Geometry check sheet. Reference: the model listing, model coordinates, mm. Coordinates: 2 decimals unless noted, no trailing zeros. Loops run counter-clockwise (first coordinate to the right, second up) from the corner with the lowest first, then second, coordinate; pieces in that order, holes last. Notation, with made-up numbers: M 79,85 L 118,85 A31 cw 118,121 Z; hole C -3,18.25 d5. An arc over 180 degrees is marked long. Use CSV: the item, a comma, the result in double quotes.
```python
from build123d import *

# Parameters (mm, degrees)
F0_R     = 11
F1_DEPTH = 6


with BuildPart() as f1:
    # F0 (on Top) → F1 (new body)
    with BuildSketch(Plane.XY):
        with BuildLine():
            ThreePointArc((36.158809, 0), (25.158809, 11), (14.158809, 0))
            ThreePointArc((14.158809, 0), (25.158809, -11), (36.158809, 0))
        make_face()
        with Locations((-25.158809, 0)):
            Circle(F0_R)
        with BuildLine():
            ThreePointArc((5.524196, 13.945725), (0, 37.658809), (-5.524196, 13.945725))
            ThreePointArc((-5.524196, 13.945725), (-8.236389, 12.536423), (-10.606602, 10.606602))
            ThreePointArc((-10.606602, 10.606602), (-12.536423, 8.236389), (-13.945725, 5.524196))
            ThreePointArc((-13.945725, 5.524196), (-37.658809, 0), (-13.945725, -5.524196))
            ThreePointArc((-13.945725, -5.524196), (-12.536423, -8.236389), (-10.606602, -10.606602))
            ThreePointArc((-10.606602, -10.606602), (-8.236389, -12.536423), (-5.524196, -13.945725))
            ThreePointArc((-5.524196, -13.945725), (0, -37.658809), (5.524196, -13.945725))
            ThreePointArc((5.524196, -13.945725), (8.236389, -12.536423), (10.606602, -10.606602))
            ThreePointArc((10.606602, -10.606602), (12.536423, -8.236389), (13.945725, -5.524196))
            ThreePointArc((13.945725, -5.524196), (37.658809, 0), (13.945725, 5.524196))
            ThreePointArc((13.945725, 5.524196), (12.536423, 8.236389), (10.606602, 10.606602))
            ThreePointArc((10.606602, 10.606602), (8.236389, 12.536423), (5.524196, 13.945725))
        make_face()
        with Locations((0, -25.158809)):
            Circle(F0_R, mode=Mode.SUBTRACT)
        with Locations((-25.158809, 0)):
            Circle(F0_R, mode=Mode.SUBTRACT)
        with BuildLine():
            ThreePointArc((-7.778175, 7.778175), (0, 11), (7.778175, 7.778175))
            ThreePointArc((7.778175, 7.778175), (10.162675, 4.209518), (11, 0))
            ThreePointArc((11, 0), (10.162675, -4.209518), (7.778175, -7.778175))
            ThreePointArc((7.778175, -7.778175), (0, -11), (-7.778175, -7.778175))
            ThreePointArc((-7.778175, -7.778175), (-10.162675, -4.209518), (-11, 0))
            ThreePointArc((-11, 0), (-10.162675, 4.209518), (-7.778175, 7.778175))
        make_face(mode=Mode.SUBTRACT)
        with BuildLine():
            ThreePointArc((36.158809, 0), (25.158809, -11), (14.158809, 0))
            ThreePointArc((14.158809, 0), (25.158809, 11), (36.158809, 0))
        make_face(mode=Mode.SUBTRACT)
        with Locations((0, 25.158809)):
            Circle(F0_R, mode=Mode.SUBTRACT)
    extrude(amount=F1_DEPTH)


solid = f1.part
```
1. Section check B-B, the plane x = 0. Record the cut outline in (y, z).
The answers:
outline,"M -37.66,0 L -36.16,0 L -36.16,6 L -37.66,6 Z; M -14.16,0 L -11,0 L -11,6 L -14.16,6 Z; M 11,0 L 14.16,0 L 14.16,6 L 11,6 Z; M 36.16,0 L 37.66,0 L 37.66,6 L 36.16,6 Z"
2. Section check A-A, the plane y = -22.5. Record the cut outline in (x, z).
The answers:
outline,"M -12.21,0 L -10.67,0 L -10.67,6 L -12.21,6 Z; M 10.67,0 L 12.21,0 L 12.21,6 L 10.67,6 Z"
3. Release check for a two-part mould opening along X. For faces 1 (the cylindrical face through (14.998, -4.213, 2.958)), 2 (the flat face through (3, -11, 0)) record: +X half, -X half, draft (parallel to the pull), parting line (faces both ways), or undercut.
The answers:
face 1,"undercut"
face 2,"draft"
4. Gauge pin test, flat ends, axial feed: P1, Ø1.5, axis at y = -21.5, z = 3.5, coming from the -X side; P2, Ø1.5, axis at y = -26, z = 4, coming from the -X side; P3, Ø13, axis at x = 0, y = -25.16, coming from the -Z side; P4, Ø8, axis at x = 9.5, y = -26, coming from the +Z side. Record the tip position at first contact, or that the pin passes through.
The answers:
P1,"x = -12.16"
P2,"x = -12.5"
P3,"through"
P4,"z = 6"
5. Section check C-C, the plane y = 2.5. Record the cut outline in (x, z), plus the area to 3 significant figures.
The answers:
outline,"M -37.41,0 L -35.87,0 L -35.87,6 L -37.41,6 Z; M -14.45,0 L -10.71,0 L -10.71,6 L -14.45,6 Z; M 10.71,0 L 14.45,0 L 14.45,6 L 10.71,6 Z; M 35.87,0 L 37.41,0 L 37.41,6 L 35.87,6 Z"
area,"63.2 mm^2"
6. Thickness scan on line 1 (Y direction, x = 0, z = 2.35); line 2 (Y direction, x = -11.5, z = 5.65); line 3 (X direction, y = -2, z = 5.6). Record the ranges inside material, lowest first. Write a range as [from, to].
The answers:
line 1,"[-37.66, -36.16], [-14.16, -11], [11, 14.16], [36.16, 37.66]"
line 2,"[-30.06, -20.26], [-9.63, 9.63], [20.26, 30.06]"
line 3,"[-37.5, -35.98], [-14.34, -10.82], [10.82, 14.34], [35.98, 37.5]"
7. Section check D-D, the plane x = -32. Record the cut outline in (y, z).
The answers:
outline,"M -10.46,0 L -8.61,0 L -8.61,6 L -10.46,6 Z; M 8.61,0 L 10.46,0 L 10.46,6 L 8.61,6 Z"
